from build123d import *

# Parameters (mm, degrees)
SKETCH_1_R      = 1.5
SKETCH_1_R_2    = 5.5
EXTRUDE_1_DEPTH = 4


with BuildPart() as part:
    # Эскиз1 → Бобышка-Вытянуть1 (new body)
    with BuildSketch(Plane.XY):
        with BuildLine():
            Line((-1.474172714, 68.016601782), (-77.746457719, 68.016601782))
            ThreePointArc((-77.746457719, 68.016601782), (-79.588811782, 68.368405195), (-81.171907265, 69.374309179))
            Line((-81.171907265, 69.374309179), (-85.184865671, 73.148357023))
            ThreePointArc((-85.184865671, 73.148357023), (-86.767961154, 74.154261006), (-88.610315217, 74.506064419))
            Line((-88.610315217, 74.506064419), (-127.610315217, 74.506064419))
            ThreePointArc((-127.610315217, 74.506064419), (-133.974276247, 71.87002545), (-136.610315217, 65.506064419))
            Line((-136.610315217, 65.506064419), (-136.610315217, 60.749014849))
            ThreePointArc((-136.610315217, 60.749014849), (-135.789339972, 56.780954297), (-133.461214308, 53.464429642))
            Line((-133.461214308, 53.464429642), (-120.803854155, 41.560622533))
            ThreePointArc((-120.803854155, 41.560622533), (-119.639791323, 39.902360205), (-119.229303701, 37.918329929))
            Line((-119.229303701, 37.918329929), (-119.229303701, -0.906201091))
            ThreePointArc((-119.229303701, -0.906201091), (-119.639791323, -2.890231366), (-120.803854155, -4.548493694))
            Line((-120.803854155, -4.548493694), (-133.461214308, -16.452300803))
            ThreePointArc((-133.461214308, -16.452300803), (-135.789339972, -19.768825459), (-136.610315217, -23.73688601))
            Line((-136.610315217, -23.73688601), (-136.610315217, -28.493935581))
            ThreePointArc((-136.610315217, -28.493935581), (-133.974276247, -34.857896611), (-127.610315217, -37.493935581))
            Line((-127.610315217, -37.493935581), (-88.610315217, -37.493935581))
            ThreePointArc((-88.610315217, -37.493935581), (-86.767961154, -37.142132167), (-85.184865671, -36.136228184))
            Line((-85.184865671, -36.136228184), (-81.171907265, -32.36218034))
            ThreePointArc((-81.171907265, -32.36218034), (-79.588811782, -31.356276357), (-77.746457719, -31.004472943))
            Line((-77.746457719, -31.004472943), (-1.474172714, -31.004472943))
            ThreePointArc((-1.474172714, -31.004472943), (0.368181349, -31.356276357), (1.951276832, -32.36218034))
            Line((1.951276832, -32.36218034), (5.964235238, -36.136228184))
            ThreePointArc((5.964235238, -36.136228184), (7.547330721, -37.142132167), (9.389684783, -37.493935581))
            Line((9.389684783, -37.493935581), (48.389684783, -37.493935581))
            ThreePointArc((48.389684783, -37.493935581), (54.753645814, -34.857896611), (57.389684783, -28.493935581))
            Line((57.389684783, -28.493935581), (57.389684783, -23.73688601))
            ThreePointArc((57.389684783, -23.73688601), (56.568709539, -19.768825459), (54.240583875, -16.452300803))
            Line((54.240583875, -16.452300803), (41.583223722, -4.548493694))
            ThreePointArc((41.583223722, -4.548493694), (40.41916089, -2.890231366), (40.008673268, -0.906201091))
            Line((40.008673268, -0.906201091), (40.008673268, 37.918329929))
            ThreePointArc((40.008673268, 37.918329929), (40.41916089, 39.902360205), (41.583223722, 41.560622533))
            Line((41.583223722, 41.560622533), (54.240583875, 53.464429642))
            ThreePointArc((54.240583875, 53.464429642), (56.568709539, 56.780954297), (57.389684783, 60.749014849))
            Line((57.389684783, 60.749014849), (57.389684783, 65.506064419))
            ThreePointArc((57.389684783, 65.506064419), (54.753645814, 71.87002545), (48.389684783, 74.506064419))
            Line((48.389684783, 74.506064419), (9.389684783, 74.506064419))
            ThreePointArc((9.389684783, 74.506064419), (7.547330721, 74.154261006), (5.964235238, 73.148357023))
            Line((5.964235238, 73.148357023), (1.951276832, 69.374309179))
            ThreePointArc((1.951276832, 69.374309179), (0.368181349, 68.368405195), (-1.474172714, 68.016601782))
        make_face()
        with Locations((-88.610315217, 69.506064419)):
            Circle(SKETCH_1_R, mode=Mode.SUBTRACT)
        with Locations((-120.610315217, 48.506064419)):
            Circle(SKETCH_1_R, mode=Mode.SUBTRACT)
        with Locations((-127.610315217, 65.506064419)):
            Circle(SKETCH_1_R_2, mode=Mode.SUBTRACT)
        with Locations((-127.610315217, -28.493935581)):
            Circle(SKETCH_1_R_2, mode=Mode.SUBTRACT)
        with Locations((-120.610315217, -11.493935581)):
            Circle(SKETCH_1_R, mode=Mode.SUBTRACT)
        with Locations((-88.610315217, -32.493935581)):
            Circle(SKETCH_1_R, mode=Mode.SUBTRACT)
        with Locations((9.389684783, -32.493935581)):
            Circle(SKETCH_1_R, mode=Mode.SUBTRACT)
        with Locations((41.389684783, -11.493935581)):
            Circle(SKETCH_1_R, mode=Mode.SUBTRACT)
        with Locations((48.389684783, -28.493935581)):
            Circle(SKETCH_1_R_2, mode=Mode.SUBTRACT)
        with Locations((48.389684783, 65.506064419)):
            Circle(SKETCH_1_R_2, mode=Mode.SUBTRACT)
        with Locations((41.389684783, 48.506064419)):
            Circle(SKETCH_1_R, mode=Mode.SUBTRACT)
        with Locations((9.389684783, 69.506064419)):
            Circle(SKETCH_1_R, mode=Mode.SUBTRACT)
    extrude(amount=EXTRUDE_1_DEPTH)


solid = part.part
For this review, take the finished solid that the model builds, in its own axes (mm). A direction names the side the tool comes from. Round coordinates to 2 decimals unless told otherwise and drop trailing zeros. Loops run counter-clockwise (first coordinate to the right, second up) from the corner with the lowest first, then second, coordinate; pieces in that order, holes last. Notation, with made-up numbers: (79.5, -32) - (114.5, -32) arc R9 cw to (114.5, -22) - close; hole circle Ø4 at (32, -30.75). An arc over 180 degrees is marked (long way). Put each result on its own line as item: value. Start each with the question number.
1. Insertion check: P1, Ø2.5, axis at x = 41.39, y = 48.51, coming from the -Z side; P2, Ø1.2, axis at y = 17, z = 2.5, coming from the +X side; P3, Ø2, axis at y = -17.5, z = 1, coming from the -X side. Each pin has a flat end and moves straight along its axis. Give the tip position at first contact, or say it passes through.
2. Consider section B-B on y = 6. State the section outline as (x, z) points.
3. Consider section A-A on x = -61. State the section outline as (y, z) points.
4. Mouldability with a two-part tool opening along X and no side actions: class faces 5 (the flat face through (-39, 68.017, 2)), 6 (the cylindrical face through (56.546, 56.729, 1.972)), 7 (the flat face through (-41, 19, 4)) as +X half, -X half, draft (parallel to the pull), parting line (faces both ways), or undercut.
5. For faces 1 (the cylindrical face through (-119.65, 39.93, 1.97)), 2 (the cylindrical face through (40.41, 39.88, 1.97)), 3 (the flat face through (-136.61, -26, 2)), 4 (the flat face through (-83.15, 71.235, 1.972)), list the 3-axis set-ups (+Z, -Z, +X, -X, +Y, -Y) from which the entire face can be reached by the end or side of a thin tool; tool diameter is ignored.
6. Consider section C-C on z = 2.55. State how many separate pieces and enclosed holes the cut face has, plus the area to 3 significant figures.
7. For probe 1 along X at (y, z) = (-29, 1.05); probe 2 along X at (y, z) = (-26.5, 2.7); probe 3 along Y at (x, z) = (-125.5, 2.7), list the stretches that pass through material, from the lowest coordinate up. Write a range as [from, to].
Result sheet:
1. P1: through
1. P2: x = 40.01
1. P3: x = -135.13
2. outline: (-119.23, 0) - (40.01, 0) - (40.01, 4) - (-119.23, 4) - close
3. outline: (-31, 0) - (68.02, 0) - (68.02, 4) - (-31, 4) - close
4. face 5: undercut
4. face 6: +X half
4. face 7: draft
5. face 1: +Z, -Z, -X
5. face 2: +Z, -Z, +X
5. face 3: +Z, -Z, -X, +Y, -Y
5. face 4: +Z, -Z, +Y
6. separate pieces: 1
6. enclosed holes: 12
6. area: 18,000 mm^2
7. probe 1: [-136.6, -133.09], [-122.13, 42.91], [53.87, 57.38]
7. probe 2: [-136.61, -132.74], [-122.48, 43.26], [53.52, 57.39]
7. probe 3: [-37.49, -33.57], [-23.41, -8.97], [45.98, 60.43], [70.59, 74.51]
